Could you check a few things on this model? Use its own coordinates, in mm. Face numbers are marked on the shaded views. A direction names the side the tool comes from. Coordinates: 2 decimals unless noted, no trailing zeros. Order: outer loops, then holes, each group sorted by start corner. A loop starts at its lowest first (then second) coordinate and runs counter-clockwise, first axis right, second up. Notation, with made-up numbers: M -33,72 L -15,72 A20 cw -15,78 Z; hole C 30.5,87.25 d10. An arc over 180 degrees is marked long. Put each result on its own line as item: value. Start each with the question number.
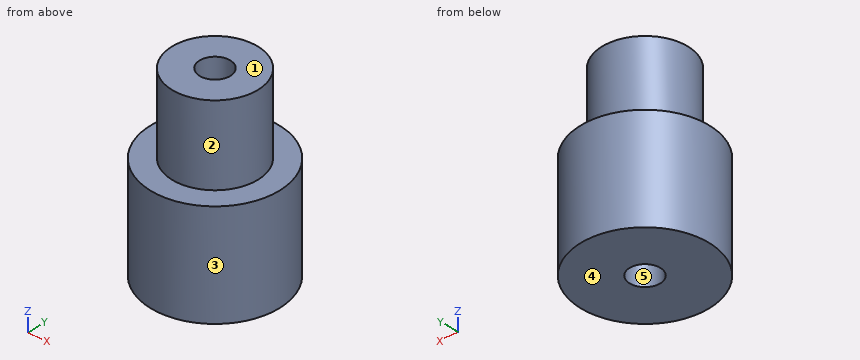
```python
from build123d import *

# Parameters (mm, degrees)
CROQUIS1_R              = 10.5
CROQUIS1_R_2            = 7
SALIENTE_EXTRUIR1_DEPTH = 17
CROQUIS2_R              = 7
SALIENTE_EXTRUIR2_DEPTH = 30
CROQUIS3_R              = 2.5
CORTAR_EXTRUIR1_DEPTH   = 58


with BuildPart() as part:
    # Croquis1 → Saliente-Extruir1 (new body)
    # profile 1 of 2: a face of its own
    with BuildSketch(Plane.XY):
        Circle(CROQUIS1_R)
        Circle(CROQUIS1_R_2, mode=Mode.SUBTRACT)
    # profile 2 of 2: a face of its own
    with BuildSketch(Plane.XY):
        Circle(CROQUIS1_R_2)
    extrude(amount=SALIENTE_EXTRUIR1_DEPTH)

    # Croquis2 → Saliente-Extruir2 (add)
    with BuildSketch(Plane.XY):
        Circle(CROQUIS2_R)
    extrude(amount=SALIENTE_EXTRUIR2_DEPTH)

    # Croquis3 → Cortar-Extruir1 (cut)
    with BuildSketch(Plane.XY):
        with Locations(Location((0, 0, 0), (0, 0, 180))):
            Circle(CROQUIS3_R)
    extrude(amount=CORTAR_EXTRUIR1_DEPTH, mode=Mode.SUBTRACT)


solid = part.part
```
Item 1: If we mould it in two halves opening along X, with no side actions, what happens to the marked faces 3, 4 and 5? For each: released by +X, released by -X, zero draft, split by the parting line, or undercut.
Item 2: For pin 1 Ø3 at (x, y) = (0, 0) entering from +Z; pin 2 Ø10 at (x, z) = (6.5, 8.5) entering from -Y; pin 3 Ø1.5 at (x, z) = (4.5, 11) entering from +Y; pin 4 Ø2 at (x, z) = (4.5, 9.5) entering from +Y, each with a flat end and sliding along its axis, tell me the tip position at first contact or that it passes through.
Item 3: For the marked faces 1 and 2, which set-ups out of +Z, -Z, +X, -X, +Y, -Y let a thin tool reach every point of the face, with its end or its side?
Item 4: If we section it at C-C on z = 11: Write out the boundary of the cut face in (x, y).
Item 5: If we section it at A-A on y = 0: Write out the boundary of the cut face in (x, z).
Item 6: I need wall thicknesses on probe 1 along Y at (x, z) = (0, 22.75); probe 2 along Y at (x, z) = (0, 14.5); probe 3 along Z at (x, y) = (-6.25, 3.25). Which ranges of each line are inside material? Lowest first, please.
Item 7: If we section it at D-D on y = -5.75: Write out the boundary of the cut face in (x, z), then the cut area to 3 significant figures.
Geometry check:
1. face 3: split by the parting line
1. face 4: zero draft
1. face 5: undercut
2. pin 1: passes through
2. pin 2: stops at y = -10.39
2. pin 3: stops at y = 9.81
2. pin 4: stops at y = 9.9
3. face 1: +Z, +X, -X, +Y, -Y
3. face 2: +Z
4. outline: C 0,0 d21; hole C 0,0 d5
5. outline: M -10.5,0 L -2.5,0 L -2.5,30 L -7,30 L -7,17 L -10.5,17 Z; M 2.5,0 L 10.5,0 L 10.5,17 L 7,17 L 7,30 L 2.5,30 Z
6. probe 1: y = -7 to -2.5, 2.5 to 7
6. probe 2: y = -10.5 to -2.5, 2.5 to 10.5
6. probe 3: z = 0 to 17
7. outline: M -8.79,0 L 8.79,0 L 8.79,17 L 3.99,17 L 3.99,30 L -3.99,30 L -3.99,17 L -8.79,17 Z
7. area: 403 mm²
